Can you work these out from the model? Positions are in its coordinate system, mm. A direction names the side the tool comes from. Round coordinates to 2 decimals unless told otherwise and drop trailing zeros. Write each loop counter-clockwise with the first axis right and the second up, starting at its lowest first coordinate (ties: lowest second). Pieces come first, ordered by that corner, then holes. Notation, with made-up numbers: M -27,63.5 L -6,63.5 A25 cw -6,87.5 Z; hole C 63.25,20 d4. An arc over 180 degrees is marked long. Answer as a JSON object with one key per item and string values. Group by question number.
1) Please list where these lines run through material, in increasing order: L1, parallel to X at y = 30, z = 10.5; L2, parallel to Y at x = 0, z = 7.5; L3, parallel to X at y = 9, z = 2.75. Write a range as [from, to].
2) On a 3-axis mill with a long thin cutter (end or side, diameter ignored), from which of +Z, -Z, +X, -X, +Y, -Y can I reach the whole of each face in a straight line? I mean faces 5 (the flat face through (5.5, -3, 7)), 6 (the flat face through (-19.31, 2.91, 6.9)), 7 (the flat face through (27.15, 49.37, 6.9)), 8 (the flat face through (21.268, 51.159, 6.902)). Say none if no direction works.
3) If we mould it in two halves opening along Y, with no side actions, what happens to faces 1 (the flat face through (-27.15, 10.63, 6.9)), 2 (the flat face through (-30, 30, 7)), 3 (the flat face through (0, 60, 7)), 4 (the flat face through (-33, 35.5, 7))? For each: +Y half, -Y half, draft (parallel to the pull), parting line (faces both ways), or undercut.
4) Suppose I cut it at C-C, the plane x = 0. Write out the boundary of the cut face in (y, z).
5) Suppose I cut it at D-D, the plane y = 11.5. Write out the boundary of the cut face in (x, z), and give its area (3 significant figures).
6) I'm going to push flat-ended pins straight in: pin 1 Ø5 at (x, z) = (12, 11.5) entering from +Y; pin 2 Ø6.5 at (x, z) = (-33.5, 9) entering from +Y; pin 3 Ø3.5 at (y, z) = (31.5, 9) entering from -X; pin 4 Ø18 at (x, y) = (0, 30) entering from +Z. Where does each tip first touch, or does it pass through?
7) Suppose I cut it at A-A, the plane y = 30. Write out the boundary of the cut face in (x, z).
from build123d import *

# Parameters (mm, degrees)
BOSS_EXTRU_1_DEPTH           = 14
ENL_V_MAT_EXTRU_1_DEPTH      = 89.577649551
ENL_V_MAT_EXTRU_1_DEPTH_BACK = 89.577649551
ESQUISSE2_R                  = 15
ESQUISSE3_R                  = 45.33486517
ESQUISSE3_R_2                = 36.129973706
ENL_V_MAT_EXTRU_2_DEPTH      = 89.577649551


with BuildPart() as part:
    # Esquisse1 → Boss.-Extru.1 (new body)
    with BuildSketch(Plane.XY):
        Polygon((-5.5, 0), (5.5, 0), (5.5, -15), (21.360912703, 0.860912703), (17.324116139, 4.897709268), (25.102290732, 12.675883861), (29.139087297, 8.639087297), (45, 24.5), (30, 24.5), (30, 35.5), (45, 35.5), (29.139087297, 51.360912703), (25.102290732, 47.324116139), (17.324116139, 55.102290732), (21.360912703, 59.139087297), (5.5, 75), (5.5, 60), (-5.5, 60), (-5.5, 75), (-21.360912703, 59.139087297), (-17.324116139, 55.102290732), (-25.102290732, 47.324116139), (-29.139087297, 51.360912703), (-45, 35.5), (-30, 35.5), (-30, 24.5), (-45, 24.5), (-29.139087297, 8.639087297), (-25.102290732, 12.675883861), (-17.324116139, 4.897709268), (-21.360912703, 0.860912703), (-5.5, -15), align=None)
    extrude(amount=BOSS_EXTRU_1_DEPTH)

    # Esquisse2 → Enlèv. mat.-Extru.1 (cut, two sides: drawn at the far end of the back side and taken through both)
    with BuildSketch(Plane.XY.offset(14).offset(-ENL_V_MAT_EXTRU_1_DEPTH_BACK)):
        with Locations((0, 30)):
            Circle(ESQUISSE2_R)
    extrude(amount=ENL_V_MAT_EXTRU_1_DEPTH + ENL_V_MAT_EXTRU_1_DEPTH_BACK, mode=Mode.SUBTRACT)

    # Esquisse3 → Enlèv. mat.-Extru.2 (cut, through all)
    with BuildSketch(Plane.XY.offset(14)):
        with Locations((0, 30)):
            Circle(ESQUISSE3_R)
        with Locations((0, 30)):
            Circle(ESQUISSE3_R_2, mode=Mode.SUBTRACT)
    extrude(amount=-ENL_V_MAT_EXTRU_2_DEPTH, mode=Mode.SUBTRACT)


solid = part.part
Results:
{
 "1": {"L1": "[-30, -15], [15, 30]", "L2": "[0, 15], [45, 60]", "L3": "[-29.4, -28.78], [-21.43, 21.43], [28.78, 29.4]"},
 "2": {"face 5": "+Z, -Z, -Y", "face 6": "+Z, -Z, -X", "face 7": "+Z, -Z, +Y", "face 8": "+Z, -Z"},
 "3": {"face 1": "-Y half", "face 2": "undercut", "face 3": "+Y half", "face 4": "undercut"},
 "4": {"outline": "M 0,0 L 15,0 L 15,14 L 0,14 Z; M 45,0 L 60,0 L 60,14 L 45,14 Z"},
 "5": {"outline": "M -31.03,0 L -26.28,0 L -26.28,14 L -31.03,14 Z; M -23.93,0 L 23.93,0 L 23.93,14 L -23.93,14 Z; M 26.28,0 L 31.03,0 L 31.03,14 L 26.28,14 Z", "area": "803 mm^2"},
 "6": {"pin 1": "y = 64.86", "pin 2": "y = 49.76", "pin 3": "x = -30", "pin 4": "through"},
 "7": {"outline": "M -30,0 L -15,0 L -15,14 L -30,14 Z; M 15,0 L 30,0 L 30,14 L 15,14 Z"}
}
